Design review of the part built by this model. Coordinates are the model's own, in mm. A direction names the side the tool comes from. Coordinates: 2 decimals unless noted, no trailing zeros. Loops run counter-clockwise (first coordinate to the right, second up) from the corner with the lowest first, then second, coordinate; pieces in that order, holes last. Notation, with made-up numbers: (-35, 69.5) - (-16, 69.5) arc R5 cw to (-16, 73.5) - close; hole circle Ø7 at (25, 65). An arc over 180 degrees is marked (long way). Return JSON: item names as keys, results as strings. Group by question number.
Autodesk Inventor part; units mm, degrees
ref_plane "YZ Plane" through (0, 0, 0) normal (1, 0, 0) x (0, 1, 0)
ref_plane "XZ Plane" through (0, 0, 0) normal (0, 1, 0) x (-1, 0, 0)
ref_plane "XY Plane" through (0, 0, 0) normal (0, 0, 1) x (1, 0, 0)
ref_plane "Work Plane3" through (-1117.6, -50.8, 0) normal (0, 0, -1) x (-1, 0, 0)
sketch "Sketch1" plane through (-1117.6, -50.8, 0) normal (0, 0, -1) x (-1, 0, 0)
  line L0 (76.5714, 45.9614) -> (29.5714, 45.9614)
  line L1 (29.5714, 45.9614) -> (29.5714, -1.0386)
  line L2 (29.5714, -1.0386) -> (76.5714, -1.0386)
  line L3 (76.5714, -1.0386) -> (76.5714, 45.9614)
  circle A0 centre (71.7603, 41.2725) radius 1
  line L4 (74.6603, 44.1725) -> (31.3603, 44.1725)
  line L5 (31.3603, 44.1725) -> (31.3603, 0.8725)
  line L6 (31.3603, 0.8725) -> (74.6603, 0.8725)
  line L7 (74.6603, 0.8725) -> (74.6603, 44.1725)
  circle A1 centre (34.2603, 41.2725) radius 1
  circle A2 centre (34.2603, 3.7725) radius 1
  circle A3 centre (71.7603, 3.7725) radius 1
  line L8 (38.6492, 8.0392) -> (67.4936, 8.0392)
  line L9 (67.4936, 8.0392) -> (67.4936, 36.8837)
  line L10 (67.4936, 36.8837) -> (38.6492, 36.8837)
  line L11 (38.6492, 36.8837) -> (38.6492, 8.0392)
  line L12 (74.6603, 0.8725) -> (68.8603, 0.8725)
  line L13 (68.8603, 0.8725) -> (68.8603, 6.6725)
  line L14 (68.8603, 6.6725) -> (74.6603, 6.6725)
  line L15 (74.6603, 6.6725) -> (74.6603, 0.8725)
  line L16 (31.3603, 0.8725) -> (37.1603, 0.8725)
  line L17 (37.1603, 0.8725) -> (37.1603, 6.6725)
  line L18 (37.1603, 6.6725) -> (31.3603, 6.6725)
  line L19 (31.3603, 6.6725) -> (31.3603, 0.8725)
  line L20 (31.3603, 44.1725) -> (37.1603, 44.1725)
  line L21 (37.1603, 44.1725) -> (37.1603, 38.3725)
  line L22 (37.1603, 38.3725) -> (31.3603, 38.3725)
  line L23 (31.3603, 38.3725) -> (31.3603, 44.1725)
  line L24 (74.6603, 44.1725) -> (68.8603, 44.1725)
  line L25 (68.8603, 44.1725) -> (68.8603, 38.3725)
  line L26 (68.8603, 38.3725) -> (74.6603, 38.3725)
  line L27 (74.6603, 38.3725) -> (74.6603, 44.1725)
  point P0 (-1117.6, 50.8)
  point P1 (53.0714, 45.9614)
  point P2 (53.0714, -1.0386)
  point P3 (31.3603, 3.7725)
  point P4 (34.2603, 44.1725)
  point P5 (31.3603, 6.6725)
  point P6 (37.1603, 0.8725)
  point P7 (74.6603, 6.6725)
  point P8 (68.8603, 0.8725)
  point P9 (74.6603, 38.3725)
  point P10 (68.8603, 44.1725)
  point P11 (31.3603, 38.3725)
  point P12 (37.1603, 44.1725)
  dimension "d1" = 47
  dimension "d2" = 47
  dimension "d4" = 2
  dimension "d6" = 1.9111
  dimension "d7" = 1.9111
  dimension "d8" = 43.3
  dimension "d9" = 43.3
  dimension "d10" = 2
  dimension "d14" = 2
  dimension "d17" = 2
  dimension "d24" = 9.0778
  dimension "d25" = 9.0778
  dimension "d26" = 9.0778
  dimension "d27" = 9.0778
  dimension "d61" = 5.8
  dimension "d62" = 5.8
  dimension "d63" = 5.8
  dimension "d64" = 5.8
  dimension "d65" = 5.8
  dimension "d66" = 5.8
  dimension "d67" = 5.8
  dimension "d68" = 5.8
  dimension "d69" = 37.5
  dimension "d70" = 37.5
  dimension "d71" = 37.5
  dimension "d72" = 37.5
  dimension "d73" = 2.9
  dimension "d74" = 2.9
extrude "Extrusion3" add sketch "Sketch1" along normal blind 8 contours L3 L2 L1 L0
extrude "Extrusion7" add sketch "Sketch1" along normal blind 3 contours L7 L26 L25 L4 | L21 L22 L5 L4 | L7 L6 L13 L14 | L18 L17 L6 L5
extrude "Extrusion8" add sketch "Sketch1" against normal blind 1 contours L3 L2 L1 L0 | A0 | L7 L26 L25 L4 | L25 L26 L7 L14 L13 L6 L17 L18 L5 L22 L21 L4 | L21 L22 L5 L4 | L7 L6 L13 L14 | L18 L17 L6 L5 | A1 | A2 | A3
extrude "Extrusion6" cut sketch "Sketch1" along normal mid plane 10 contours A0 | A1 | A2 | A3
fillet "Fillet5" radius 10 4 edges at (-1156.2492, -13.9163, 0.5) (-1185.0936, -13.9163, 0.5) (-1185.0936, -42.7608, 0.5) (-1156.2492, -42.7608, 0.5)
fillet "Fillet6" radius 2 4 edges at (-1194.1714, -4.8386, -3.5) (-1147.1714, -4.8386, -3.5) (-1194.1714, -51.8386, -3.5) (-1147.1714, -51.8386, -3.5)
fillet "Fillet7" radius 4 4 edges at (-1154.7603, -12.4275, -1.5) (-1186.4603, -12.4275, -1.5) (-1186.4603, -44.1275, -1.5) (-1154.7603, -44.1275, -1.5)
equation "\"d10\" = d4"
equation "\"d14\" = d4"
equation "\"d17\" = d4"
equation "\"d61\" = 2 * d73"
equation "\"d73\" = -0.5 * d72 + 0.5 * d8"
properties part number "bracket"
Item 1: Add section C-C (z = -6.75). State the section outline as (x, y) points, then the cut area to 3 significant figures.
Item 2: Add section B-B (y = -29). State the section outline as (x, z) points, then the cut area to 3 significant figures.
Item 3: Add section A-A (x = -1168). State the section outline as (y, z) points, then the cut area to 3 significant figures.
Item 4: For faces 5 (the face through (-1187.66, -45.27, -1.52)), 6 (the face through (-1182.242, -39.754, 0.507)), 7 (the face through (-1169, -51, -8)), list the 3-axis set-ups (+Z, -Z, +X, -X, +Y, -Y) from which the entire face can be reached by the end or side of a thin tool; tool diameter is ignored.
Item 5: For P1, Ø8, axis at x = -1157.5, y = -34, coming from the -Z side; P2, Ø4.5, axis at x = -1150.5, y = -46.5, coming from the -Z side; P3, Ø4.5, axis at x = -1189, y = -46, coming from the -Z side, all flat-tipped, find the tip position at first contact; note any pin that passes through.
Item 6: To check wall thickness, follow line 1 (X direction, y = -7.5, z = -4.5); line 2 (Y direction, x = -1160, z = -7.25); line 3 (X direction, y = -9, z = -1). State the ranges of each line that lie inside material, in increasing order. Write a range as from..to.
Item 7: Add section D-D (z = -2.25). State the section outline as (x, y) points.
Item 8: Draft analysis for pull direction Y (two halves, no side actions). For faces 1 (the face through (-1153.62, -45.33, -1.52)), 2 (the face through (-1147.77, -5.41, -3.56)), 3 (the face through (-1170, -51.839, -3)), 4 (the face through (-1190.314, -46.727, -1.028)), state which applies: pulls with the +Y half, pulls with the -Y half, needs draft (parallel to the pull), parting line crosses it, or undercut.
Answers below:
{
 "1": {"outline": "(-1194.17, -49.84) arc R2 ccw to (-1192.17, -51.84) - (-1149.17, -51.84) arc R2 ccw to (-1147.17, -49.84) - (-1147.17, -6.84) arc R2 ccw to (-1149.17, -4.84) - (-1192.17, -4.84) arc R2 ccw to (-1194.17, -6.84) - close; hole (-1192.26, -49.93) - (-1148.96, -49.93) - (-1148.96, -6.63) - (-1192.26, -6.63) - close", "area": "331 mm^2"},
 "2": {"outline": "(-1194.17, -8) - (-1192.26, -8) - (-1192.26, 0) - (-1185.09, 0) - (-1185.09, 1) - (-1194.17, 1) - close; (-1156.25, 0) - (-1148.96, 0) - (-1148.96, -8) - (-1147.17, -8) - (-1147.17, 1) - (-1156.25, 1) - close", "area": "47.8 mm^2"},
 "3": {"outline": "(-51.84, -8) - (-49.93, -8) - (-49.93, 0) - (-42.76, 0) - (-42.76, 1) - (-51.84, 1) - close; (-13.92, 0) - (-6.63, 0) - (-6.63, -8) - (-4.84, -8) - (-4.84, 1) - (-13.92, 1) - close", "area": "47.8 mm^2"},
 "4": {"face 5": "-Z", "face 6": "+Z, -Z", "face 7": "-Z, +X, -X, +Y, -Y"},
 "5": {"P1": "stops at z = 0", "P2": "stops at z = -8", "P3": "stops at z = -3"},
 "6": {"line 1": "x = -1194.17..-1192.26, -1148.96..-1147.17", "line 2": "y = -51.84..-49.93, -6.63..-4.84", "line 3": "x = -1194.17..-1190.21, -1188.51..-1186.5, -1154.72..-1152.71, -1151.01..-1147.17"},
 "7": {"outline": "(-1194.17, -49.84) arc R2 ccw to (-1192.17, -51.84) - (-1149.17, -51.84) arc R2 ccw to (-1147.17, -49.84) - (-1147.17, -6.84) arc R2 ccw to (-1149.17, -4.84) - (-1192.17, -4.84) arc R2 ccw to (-1194.17, -6.84) - close; hole (-1192.26, -44.13) - (-1190.46, -44.13) arc R4 cw to (-1186.46, -48.13) - (-1186.46, -49.93) - (-1154.76, -49.93) - (-1154.76, -48.13) arc R4 cw to (-1150.76, -44.13) - (-1148.96, -44.13) - (-1148.96, -12.43) - (-1150.76, -12.43) arc R4 cw to (-1154.76, -8.43) - (-1154.76, -6.63) - (-1186.46, -6.63) - (-1186.46, -8.43) arc R4 cw to (-1190.46, -12.43) - (-1192.26, -12.43) - close; hole circle Ø2 at (-1189.36, -47.03); hole circle Ø2 at (-1189.36, -9.53); hole circle Ø2 at (-1151.86, -47.03); hole circle Ø2 at (-1151.86, -9.53)"},
 "8": {"face 1": "undercut", "face 2": "pulls with the +Y half", "face 3": "pulls with the -Y half", "face 4": "undercut"}
}
